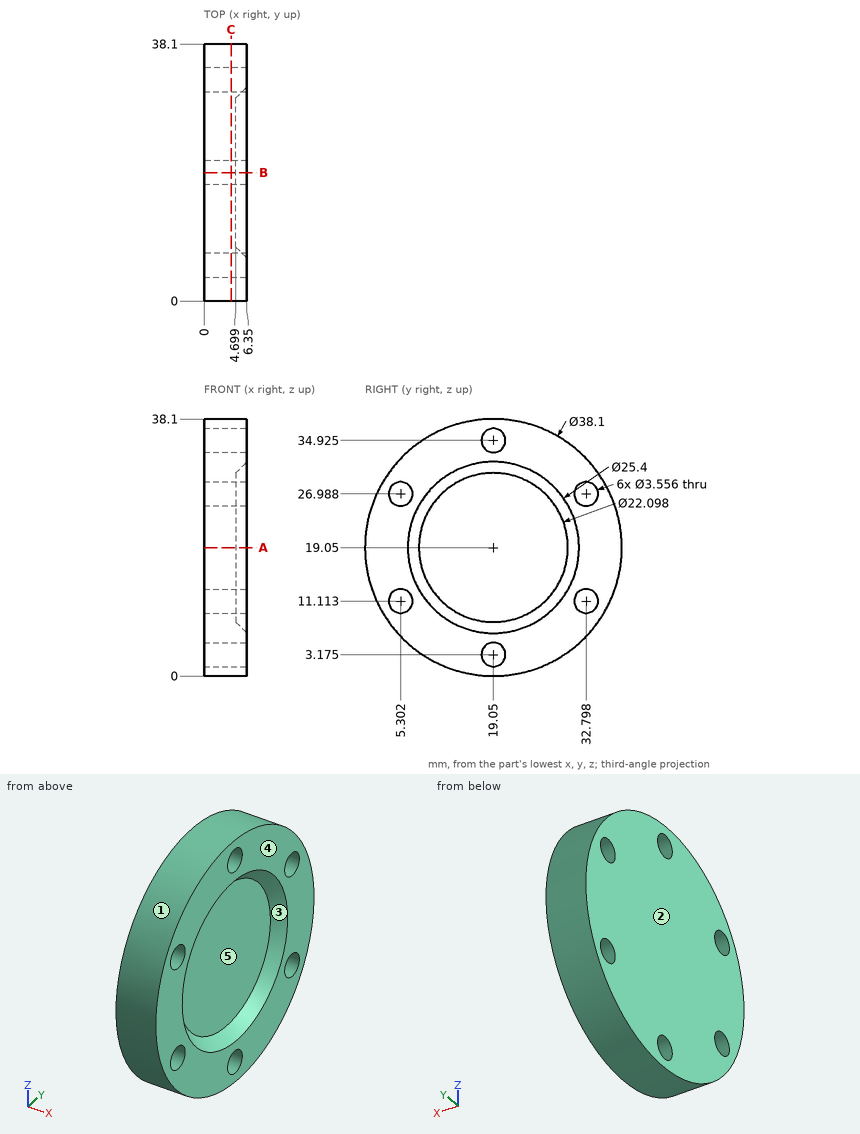
Design review of the part shown in the three views and the two pictorial views. Dimensions are in mm from the part's minimum x, y and z. A direction names the side the tool comes from. Give positions to 0.01 mm unless a question says otherwise; leave off trailing zeros. Loops run counter-clockwise (first coordinate to the right, second up) from the corner with the lowest first, then second, coordinate; pieces in that order, holes last. Notation, with made-up numbers: (3.5, -11) -> (56.5, -11) arc R22 cw to (56.5, 18) -> close; hole circle Ø5 at (18.5, -24). An arc over 180 degrees is marked (long way). Answer as a JSON object with one key per item and string values. Group by question number.
Q1. Insertion check: pin 1 (1.5 mm diameter, centred on x = 5, y = 7, fed in from +Z); pin 2 (3 mm diameter, centred on y = 32.8, z = 26.99, fed in from -X); pin 3 (6.5 mm diameter, centred on y = 23, z = 17, fed in from +X). Each pin has a flat end and moves straight along its axis. Give the tip position at first contact, or say it passes through.
Q2. Wall thickness on line 1 along Z through (x, y) = (3.5, 19); line 2 along Z through (x, y) = (1, 18); line 3 along Y through (x, z) = (3.25, 19): over which ranges is each line inside the solid? List them lowest first.
Q3. Take a section at B-B (y = 19.05). Write out the cut boundary in (x, z).
Q4. Take a section at C-C (x = 4). State how many separate pieces and enclosed holes the cut face has, plus the area to 3 significant figures.
Q5. Draft analysis for pull direction Z (two halves, no side actions). For the marked faces 1, 2 and 3, state which applies: pulls with the +Z half, pulls with the -Z half, needs draft (parallel to the pull), parting line crosses it, or undercut.
Q6. Tool access review of the marked faces 4 and 5: name each direction out of +Z, -Z, +X, -X, +Y, -Y from which nothing blocks a thin tool from reaching the whole face with its end or side.
Q7. Take a section at A-A (z = 19.05). Write out the cut boundary in (x, y).
Answer below:
{
 "1": {"pin 1": "stops at z = 34.39", "pin 2": "passes through", "pin 3": "stops at x = 4.7"},
 "2": {"line 1": "z = 0 to 1.4, 4.95 to 33.15, 36.7 to 38.1", "line 2": "z = 0.03 to 1.74, 4.61 to 33.49, 36.36 to 38.07", "line 3": "y = 0 to 38.1"},
 "3": {"outline": "(0, 0) -> (6.35, 0) -> (6.35, 1.4) -> (0, 1.4) -> close; (0, 4.95) -> (6.35, 4.95) -> (6.35, 6.35) -> (4.7, 8) -> (4.7, 30.1) -> (6.35, 31.75) -> (6.35, 33.15) -> (0, 33.15) -> close; (0, 36.7) -> (6.35, 36.7) -> (6.35, 38.1) -> (0, 38.1) -> close"},
 "4": {"separate pieces": "1", "enclosed holes": "6", "area": "1,080 mm2"},
 "5": {"face 1": "parting line crosses it", "face 2": "needs draft", "face 3": "undercut"},
 "6": {"face 4": "+Z, -Z, +X, +Y, -Y", "face 5": "+X"},
 "7": {"outline": "(0, 0) -> (6.35, 0) -> (6.35, 6.35) -> (4.7, 8) -> (4.7, 30.1) -> (6.35, 31.75) -> (6.35, 38.1) -> (0, 38.1) -> close"}
}
